```python
from build123d import *

# Parameters (mm, degrees)
ESBO_O1_W                   = 56
ESBO_O1_H                   = 76
RESSALTO_EXTRUS_O1_DEPTH    = 2
ESBO_O1_3_W                 = 56
ESBO_O1_3_H                 = 76
ESBO_O1_3_W_2               = 52
ESBO_O1_3_H_2               = 72
RESSALTO_EXTRUS_O2_DEPTH    = 18
ESBO_O2_R                   = 2.5
ESBO_O2_R_2                 = 1
RESSALTO_EXTRUS_O3_DEPTH    = 3.5
ESPELHAR2_COPY_1_SKETCH_R   = 2.5
ESPELHAR2_COPY_1_SKETCH_R_2 = 1
ESPELHAR2_COPY_1_DEPTH      = 3.5
ESBO_O3_R                   = 1.25
CORTE_EXTRUS_O1_DEPTH       = 83.969874051


with BuildPart() as part:
    # Esbo_o1 → Ressalto-extrus_o1 (new body)
    with BuildSketch(Plane.XY):
        Rectangle(ESBO_O1_W, ESBO_O1_H)
    extrude(amount=-RESSALTO_EXTRUS_O1_DEPTH)

    # Esbo_o1_3 → Ressalto-extrus_o2 (add)
    with BuildSketch(Plane.XY):
        Rectangle(ESBO_O1_3_W, ESBO_O1_3_H)
        Rectangle(ESBO_O1_3_W_2, ESBO_O1_3_H_2, mode=Mode.SUBTRACT)
    extrude(amount=RESSALTO_EXTRUS_O2_DEPTH)

    # Esbo_o2 → Ressalto-extrus_o3 (add)
    # profile 1 of 2: a face of its own
    with BuildSketch(Plane.XY):
        with Locations((-23, 33)):
            Circle(ESBO_O2_R)
        with Locations((-23, 33)):
            Circle(ESBO_O2_R_2, mode=Mode.SUBTRACT)
    # profile 2 of 2: a face of its own
    with BuildSketch(Plane.XY):
        with BuildLine():
            ThreePointArc((-23, 30.5), (-24.767766953, 34.767766953), (-20.5, 33))
            Line((-20.5, 33), (-20.5, 36))
            Line((-20.5, 36), (-26, 36))
            Line((-26, 36), (-26, 30.5))
            Line((-26, 30.5), (-23, 30.5))
        make_face()
    ressalto_extrus_o3 = extrude(amount=RESSALTO_EXTRUS_O3_DEPTH)

    # Espelhar1: Ressalto-extrus_o3 across plane
    add(ressalto_extrus_o3.mirror(Plane(origin=(0, 0, 0), x_dir=(0, 0, 1), z_dir=(1, 0, 0))))

    # Espelhar2: Ressalto-extrus_o3 across plane
    add(ressalto_extrus_o3.mirror(Plane.ZX))

    # Espelhar2 copy 1 sketch → Espelhar2 copy 1 (add)
    # profile 1 of 2: a face of its own
    with BuildSketch(Plane(origin=(0, 0, 0), x_dir=(-1, 0, 0), z_dir=(0, 0, 1))):
        with Locations((-23, 33)):
            Circle(ESPELHAR2_COPY_1_SKETCH_R)
        with Locations((-23, 33)):
            Circle(ESPELHAR2_COPY_1_SKETCH_R_2, mode=Mode.SUBTRACT)
    # profile 2 of 2: a face of its own
    with BuildSketch(Plane(origin=(0, 0, 0), x_dir=(-1, 0, 0), z_dir=(0, 0, 1))):
        with BuildLine():
            ThreePointArc((-23, 30.5), (-24.767766953, 34.767766953), (-20.5, 33))
            Line((-20.5, 33), (-20.5, 36))
            Line((-20.5, 36), (-26, 36))
            Line((-26, 36), (-26, 30.5))
            Line((-26, 30.5), (-23, 30.5))
        make_face()
    extrude(amount=ESPELHAR2_COPY_1_DEPTH)

    # Esbo_o3 → Corte-extrus_o1 (cut, through all)
    with BuildSketch(Plane.XZ.offset(38)):
        with Locations(Location((-22, 15, 0), (0, 0, 270))):
            Circle(ESBO_O3_R)
        with Locations(Location((22, 15, 0), (0, 0, 90))):
            Circle(ESBO_O3_R)
    extrude(amount=-CORTE_EXTRUS_O1_DEPTH, mode=Mode.SUBTRACT)


solid = part.part
```
Geometry check sheet. Reference: the model listing, model coordinates, mm. A direction names the side the tool comes from. Round coordinates to 2 decimals unless told otherwise and drop trailing zeros. Order: outer loops, then holes, each group sorted by start corner. A loop starts at its lowest first (then second) coordinate and runs counter-clockwise, first axis right, second up. Notation, with made-up numbers: (69, 86) - (81, 86) arc R24 ccw to (81, 110) - close; hole circle Ø5 at (41, 21.25). An arc over 180 degrees is marked (long way). Use a Markdown table: item, result. Add a question column.
1) Thickness scan on line 1 along X through (y, z) = (-33, 2.6); line 2 along X through (y, z) = (36.85, 15); line 3 along Y through (x, z) = (-23, 1.45). Record the ranges inside material, lowest first.
2) Mould release check, pull along Y, two halves, no side actions. Record for faces 1 (the flat face through (0, 38, 8)), 2 (the flat face through (-20.5, 34, 2)), 3 (the flat face through (0, 1, -2)): released by +Y, released by -Y, zero draft, split by the parting line, or undercut.
3) Section check D-D (x = 13.5). Record the cut outline in (y, z), then the cut area to 3 significant figures.
4) Set-up check for faces 4 (the flat face through (0, 36, 9)), 5 (the cylindrical face through (23.22, -37.01, 14.73)): record each of +Z, -Z, +X, -X, +Y, -Y from which the full face is reachable in a straight line by a thin tool's end or side.
5) Section check A-A (z = 15). Record the cut outline in (x, y).
6) Section check C-C (z = 11.5). Record the cut outline in (x, y), then the cut area to 3 significant figures.
7) Gauge pin test, flat ends, axial feed: P1, Ø2, axis at x = 22, z = 15, coming from the +Y side; P2, Ø2, axis at x = 10, y = 1.5, coming from the +Z side; P3, Ø4.5, axis at x = -23.5, y = -32.5, coming from the +Z side. Record the tip position at first contact, or that the pin passes through.
8) Section check B-B (y = -11). Record the cut outline in (x, z).
Established:
| question | item | result |
|---|---|---|
| 1 | line 1 | -28 to -24, -22 to -20.5, 20.5 to 22, 24 to 28 |
| 1 | line 2 | -28 to -23.25, -20.75 to 20.75, 23.25 to 28 |
| 1 | line 3 | -38 to -34, -32 to -30.5, 30.5 to 32, 34 to 38 |
| 2 | face 1 | released by +Y |
| 2 | face 2 | undercut |
| 2 | face 3 | zero draft |
| 3 | outline | (-38, -2) - (38, -2) - (38, 18) - (36, 18) - (36, 0) - (-36, 0) - (-36, 18) - (-38, 18) - close |
| 3 | area | 224 mm2 |
| 4 | face 4 | +Z |
| 4 | face 5 | +Y, -Y |
| 5 | outline | (-28, -38) - (-23.25, -38) - (-23.25, -36) - (-26, -36) - (-26, 36) - (-23.25, 36) - (-23.25, 38) - (-28, 38) - close; (-20.75, -38) - (20.75, -38) - (20.75, -36) - (-20.75, -36) - close; (-20.75, 36) - (20.75, 36) - (20.75, 38) - (-20.75, 38) - close; (23.25, -38) - (28, -38) - (28, 38) - (23.25, 38) - (23.25, 36) - (26, 36) - (26, -36) - (23.25, -36) - close |
| 6 | outline | (-28, -38) - (28, -38) - (28, 38) - (-28, 38) - close; hole (-26, -36) - (26, -36) - (26, 36) - (-26, 36) - close |
| 6 | area | 512 mm2 |
| 7 | P1 | through |
| 7 | P2 | z = 0 |
| 7 | P3 | z = 3.5 |
| 8 | outline | (-28, -2) - (28, -2) - (28, 18) - (26, 18) - (26, 0) - (-26, 0) - (-26, 18) - (-28, 18) - close |
